Could you check a few things on this model? Use its own coordinates, in mm. A direction names the side the tool comes from. Round coordinates to 2 decimals unless told otherwise and drop trailing zeros. Write each loop counter-clockwise with the first axis right and the second up, starting at its lowest first coordinate (ties: lowest second). Pieces come first, ordered by that corner, then holes. Notation, with made-up numbers: (-30, -37) -> (1, -37) arc R35 cw to (1, -4) -> close; hole circle Ø4 at (-21.75, -38.5). An arc over 180 degrees is marked (long way). Return JSON: item names as keys, results as strings.
from build123d import *

# Parameters (mm, degrees)
SKETCH1_R           = 14
SKETCH1_R_2         = 19
SKETCH1_R_3         = 6
BOSS_EXTRUDE1_DEPTH = 12
FILLET1_R           = 50


with BuildPart() as part:
    # Sketch1 → Boss-Extrude1 (new body)
    with BuildSketch(Plane(origin=(0, 0, 0), x_dir=(1, 0, 0), z_dir=(0, 1, 0))):
        with BuildLine():
            Line((31.065401992, 0), (18.389205605, 48.778819646))
            ThreePointArc((18.389205605, 48.778819646), (18.846682818, 46.408847598), (19, 44))
            ThreePointArc((19, 44), (-2.385148225, 25.15030324), (-18.401165047, 48.732560082))
            Line((-18.401165047, 48.732560082), (-30.934598008, 0))
            Line((-30.934598008, 0), (-18.401165047, -48.732560082))
            ThreePointArc((-18.401165047, -48.732560082), (-2.385148225, -25.15030324), (19, -44))
            ThreePointArc((19, -44), (18.846682818, -46.408847598), (18.389205605, -48.778819646))
            Line((18.389205605, -48.778819646), (31.065401992, 0))
        make_face()
        Circle(SKETCH1_R, mode=Mode.SUBTRACT)
        with Locations((0, -44)):
            Circle(SKETCH1_R_2)
        with Locations((0, -44)):
            Circle(SKETCH1_R_3, mode=Mode.SUBTRACT)
        with Locations((0, 44)):
            Circle(SKETCH1_R_2)
        with Locations((0, 44)):
            Circle(SKETCH1_R_3, mode=Mode.SUBTRACT)
    extrude(amount=BOSS_EXTRUDE1_DEPTH)

    # Fillet1
    fillet1_edges = [part.edges().sort_by_distance(p)[0] for p in [
        (-30.934598008, 6, 0),
        (31.065401992, 6, 0),
    ]]
    fillet(fillet1_edges, radius=FILLET1_R)

    # Sketch3 → Revolve1 (revolve)
    with BuildSketch(Plane.XY):
        Polygon((14, 0), (28, 0), (28, -30), (14, -21.917096231), align=None)
    revolve(axis=Axis((0, 0, 0), (0, -1, 0)))


solid = part.part
1) I want a section at D-D, the plane y = -10.5. Please give me the cut outline in (x, z).
Return value:
{"outline": "circle Ø56 at (0, 0); hole circle Ø28 at (0, 0)"}
2) If I drill on probe 1 along Z at (x, y) = (0, 5.25); probe 2 along Z at (x, y) = (0, -15); probe 3 along X at (y, z) = (1, 0), over which ranges is the centre line in solid material (lowest first)? Write a range as [from, to].
Return value:
{"probe 1": "[-63, -50], [-38, -14], [14, 38], [50, 63]", "probe 2": "[-28, -14], [14, 28]", "probe 3": "[-29.31, -14], [14, 29.4]"}
3) Thinking about a two-plate mould opening in Z: for faces 3 (the face through (-29.307, 6.084, -0.176)), 4 (the face through (-1.301, 5.916, 49.857)), 5 (the face through (-23, 5.92, -30.85)), which applies, pulls with the +Z half, pulls with the -Z half, needs draft (parallel to the pull), parting line crosses it, or undercut?
Return value:
{"face 3": "parting line crosses it", "face 4": "undercut", "face 5": "pulls with the -Z half"}
4) I want a section at C-C, the plane z = -44. Please give me the cut outline in (x, y), and give its area (3 significant figures).
Return value:
{"outline": "(-19.62, 0) -> (-6, 0) -> (-6, 12) -> (-19.62, 12) -> close; (6, 0) -> (19.63, 0) -> (19.63, 12) -> (6, 12) -> close", "area": "327 mm²"}
5) I want a section at B-B, the plane y = 5. Please give me the cut outline in (x, z).
Return value:
{"outline": "(-27.73, -12.45) -> (-18.4, -48.73) arc R19 ccw to (18.39, -48.78) -> (27.8, -12.58) arc R50 ccw to (27.8, 12.58) -> (18.39, 48.78) arc R19 ccw to (-18.4, 48.73) -> (-27.73, 12.45) arc R50 ccw to start; hole circle Ø28 at (0, 0); hole circle Ø12 at (0, -44); hole circle Ø12 at (0, 44)"}
6) I want a section at A-A, the plane z = 0. Please give me the cut outline in (x, y), and give its area (3 significant figures).
Return value:
{"outline": "(-29.31, 0) -> (-28, 0) -> (-28, -30) -> (-14, -21.92) -> (-14, 12) -> (-29.31, 12) -> close; (14, -21.92) -> (28, -30) -> (28, 0) -> (29.4, 0) -> (29.4, 12) -> (14, 12) -> close", "area": "1,100 mm²"}
7) For faces 1 (the face through (12.932, -4.721, -5.362)), 2 (the face through (25.865, -15.21, -10.724)), which set-ups out of +Z, -Z, +X, -X, +Y, -Y let a thin tool reach every point of the face, with its end or its side?
Return value:
{"face 1": "+Y, -Y", "face 2": "-Y"}
8) Will these pins go through, and if not, where does the flat tip stop? pin 1 Ø1 at (x, z) = (-23.5, -11.5) entering from -Y; pin 2 Ø6 at (x, y) = (-6.5, -9) entering from -Z; pin 3 Ø1.5 at (x, y) = (1.5, -6.5) entering from +Z.
Return value:
{"pin 1": "y = -29.23", "pin 2": "z = -27.78", "pin 3": "z = 27.99"}
